Here's how the part is built. I have some questions about the finished solid (model axes, mm). A direction names the side the tool comes from. Round coordinates to 2 decimals unless told otherwise and drop trailing zeros. Order: outer loops, then holes, each group sorted by start corner. A loop starts at its lowest first (then second) coordinate and runs counter-clockwise, first axis right, second up. Notation, with made-up numbers: M -26.5,80.25 L 17.5,80.25 A30 cw 17.5,112.25 Z; hole C -1.5,47 d1. An arc over 180 degrees is marked long. Write item = value, one per line. Start each with the question number.
Item 1: For faces 1 (the face through (-8.075, 12, 17)), 2 (the face through (-0.553, 7.605, 30.742)), 3 (the face through (0, 27, 10)), which set-ups out of +Z, -Z, +X, -X, +Y, -Y let a thin tool reach every point of the face, with its end or its side?
Item 2: I want a section at B-B, the plane z = 13. List the corners of the cut face in (x, y) for me, plus the area to 3 significant figures.
Item 3: I want a section at D-D, the plane y = 18.25. List the corners of the cut face in (x, z) for me, plus the area to 3 significant figures.
Item 4: I want a section at A-A, the plane y = 26. List the corners of the cut face in (x, z) for me.
Item 5: I'm going to push flat-ended pins straight in: P1, Ø3, axis at x = -7, z = 7.5, coming from the +Y side; P2, Ø1.5, axis at x = 2.5, y = 27, coming from the -Z side; P3, Ø4, axis at y = 13, z = 23, coming from the -X side. Where does each tip first touch, or does it pass through?
Item 6: We'd pull the mould along X, two halves only. Please class faces 4 (the face through (-0.553, 7.605, 10.742)), 5 (the face through (0, 25.133, 27)), 6 (the face through (-9.35, 26.86, 22.34)): pulls with the +X half, pulls with the -X half, needs draft (parallel to the pull), parting line crosses it, or undercut.
Item 7: Please list where these lines run through material, in increasing order: L1, parallel to Z at x = 0, y = 5.25; L2, parallel to Z at x = -0.5, y = 26; L3, parallel to X at y = 8.75, z = 28.25.
Item 8: I want a section at C-C, the plane x = -6.5. List the corners of the cut face in (y, z) for me, plus the area to 3 significant figures.
```python
from build123d import *

# Parameters (mm, degrees)
BOSS_EXTRUDE1_DEPTH         = 35.25
F_1_4_20_TAPPED_HOLE1_D     = 5.1054
F_1_4_20_TAPPED_HOLE1_DEPTH = 15
F_1_4_20_TAPPED_HOLE1_TIP   = 1.533816902
SKETCH4_W                   = 6.24022781
SKETCH4_H                   = 5.25
SKETCH4_W_2                 = 16.14963906
SKETCH4_W_3                 = 28.63009468
CUT_EXTRUDE1_DEPTH          = 3


with BuildPart() as part:
    # Sketch1 → Boss-Extrude1 (new body)
    with BuildSketch(Plane.XY):
        Polygon((-8.07481953, 0), (8.07481953, 0), (8.07481953, 22.9672), (10.65761953, 25.55), (8.07481953, 28.1328), (-8.07481953, 28.1328), (-10.65761953, 25.55), (-8.07481953, 22.9672), align=None)
    extrude(amount=BOSS_EXTRUDE1_DEPTH)

    # 1/4-20 Tapped Hole1
    with Locations(Plane(origin=(0, 0, 0), x_dir=(-1, 0, 0), z_dir=(0, -1, 0))):
        with Locations((0, -8.25), (0, -28.25)):
            Hole(F_1_4_20_TAPPED_HOLE1_D / 2, depth=F_1_4_20_TAPPED_HOLE1_DEPTH)
            with Locations((0, 0, -(F_1_4_20_TAPPED_HOLE1_DEPTH + F_1_4_20_TAPPED_HOLE1_TIP / 2))):  # 118° drill point
                Cone(0, F_1_4_20_TAPPED_HOLE1_D / 2, F_1_4_20_TAPPED_HOLE1_TIP, mode=Mode.SUBTRACT)

    # Sketch4 → Cut-Extrude1 (cut)
    with BuildSketch(Plane(origin=(0, 28.1328, 0), x_dir=(1, 0, 0), z_dir=(0, 1, 0))):
        with Locations((-11.194933435, -17.375)):
            Rectangle(SKETCH4_W, SKETCH4_H)
        with Locations((0, -17.375)):
            Rectangle(SKETCH4_W_2, SKETCH4_H)
        with Locations((11.194933435, -17.375)):
            Rectangle(SKETCH4_W, SKETCH4_H)
        with Locations((-11.194933435, -27.375)):
            Rectangle(SKETCH4_W, SKETCH4_H)
        with Locations((0, -27.375)):
            Rectangle(SKETCH4_W_2, SKETCH4_H)
        with Locations((11.194933435, -27.375)):
            Rectangle(SKETCH4_W, SKETCH4_H)
        with Locations((0, -7.375)):
            Rectangle(SKETCH4_W_3, SKETCH4_H)
    extrude(amount=-CUT_EXTRUDE1_DEPTH, mode=Mode.SUBTRACT)


solid = part.part
```
Filled in:
q1.face_1 = +Z, -Z, -X, -Y
q1.face_2 = -Y
q1.face_3 = +X, -X, +Y
q2.outline = M -10.66,25.55 L -8.07,22.97 L -8.07,0 L 8.07,0 L 8.07,22.97 L 10.66,25.55 L 8.07,28.13 L -8.07,28.13 Z
q2.area = 468 mm^2
q3.outline = M -8.07,0 L 8.07,0 L 8.07,35.25 L -8.07,35.25 Z
q3.area = 569 mm^2
q4.outline = M -10.21,0 L 10.21,0 L 10.21,4.75 L -10.21,4.75 Z; M -10.21,10 L 10.21,10 L 10.21,14.75 L -10.21,14.75 Z; M -10.21,20 L 10.21,20 L 10.21,24.75 L -10.21,24.75 Z; M -10.21,30 L 10.21,30 L 10.21,35.25 L -10.21,35.25 Z
q5.P1 = 25.13
q5.P2 = 0
q5.P3 = -8.07
q6.face_4 = undercut
q6.face_5 = needs draft
q6.face_6 = pulls with the -X half
q7.L1 = 0 to 5.7, 10.8 to 25.7, 30.8 to 35.25
q7.L2 = 0 to 4.75, 10 to 14.75, 20 to 24.75, 30 to 35.25
q7.L3 = -8.07 to -2.55, 2.55 to 8.07
q8.outline = M 0,0 L 28.13,0 L 28.13,4.75 L 25.13,4.75 L 25.13,10 L 28.13,10 L 28.13,14.75 L 25.13,14.75 L 25.13,20 L 28.13,20 L 28.13,24.75 L 25.13,24.75 L 25.13,30 L 28.13,30 L 28.13,35.25 L 0,35.25 Z
q8.area = 944 mm^2
